Can you work these out from the model? Positions are in its coordinate system, mm. A direction names the side the tool comes from. Give positions to 0.01 mm unless a question says otherwise; leave off trailing zeros. Loops run counter-clockwise (first coordinate to the right, second up) from the corner with the lowest first, then second, coordinate; pieces in that order, holes last. Notation, with made-up numbers: (86, -14) - (129, -14) arc R13 cw to (129, 3) - close; hole circle Ø11 at (17.5, 57). An arc over 180 degrees is marked (long way). Answer as a JSON object with one key per item and string values.
```python
from build123d import *

# Parameters (mm, degrees)
IZIM1_W                     = 10
IZIM1_H                     = 20
Y_KSEKLIK_EKSTR_ZYON1_DEPTH = 150
BO_ALTMA1_T                 = -1
IZIM4_R                     = 2
KES_EKSTR_ZYON3_DEPTH       = 18


with BuildPart() as part:
    # Çizim1 → Yükseklik-Ekstrüzyon1 (new, symmetric)
    with BuildSketch(Plane.XY):
        Rectangle(IZIM1_W, IZIM1_H)
    extrude(amount=Y_KSEKLIK_EKSTR_ZYON1_DEPTH, both=True)

    # İç Boşaltma1
    bo_altma1_openings = [part.faces().sort_by_distance(p)[0] for p in [
        (0, 0, 150),
    ]]
    offset(amount=BO_ALTMA1_T, openings=bo_altma1_openings, kind=Kind.INTERSECTION)

    # Çizim4 → Kes-Ekstrüzyon3 (cut)
    with BuildSketch(Plane(origin=(5, 0, 0), x_dir=(0, 0, -1), z_dir=(1, 0, 0))):
        with Locations(Location((-99.95519869, 6.5, 0), (0, 0, 90))):
            Circle(IZIM4_R)
        with Locations(Location((-99.95519869, -6.5, 0), (0, 0, 90))):
            Circle(IZIM4_R)
    extrude(amount=-KES_EKSTR_ZYON3_DEPTH, mode=Mode.SUBTRACT)


solid = part.part
```
1) I'm going to push a flat-ended pin straight in: P1, Ø3.5, axis at y = 6.5, z = 99.96, coming from the +X side. Where does the tip first touch, or does it pass through?
Check sheet entries:
{"P1": "through"}
2) I need wall thicknesses on L1, parallel to Y at x = -0.25, z = -32.5; L2, parallel to X at y = -6.75, z = -80.5; L3, parallel to Z at x = 4.5, y = -6.5. Which ranges of each line are inside material? Lowest first, please.
Check sheet entries:
{"L1": "-10 to -9, 9 to 10", "L2": "-5 to -4, 4 to 5", "L3": "-150 to 97.96, 101.96 to 150"}
3) Imagine slicing it at A-A on x = -1.75. Write out the boundary of the cut face in (y, z), and give its area (3 significant figures).
Check sheet entries:
{"outline": "(-10, -150) - (10, -150) - (10, 150) - (9, 150) - (9, -149) - (-9, -149) - (-9, 150) - (-10, 150) - close", "area": "618 mm2"}
4) If we mould it in two halves opening along Y, with no side actions, what happens to faces 3 (the flat face through (0, 0, -150)), 4 (the flat face through (-4, 0, 3)), 5 (the flat face through (0, 9, 3)), 6 (the flat face through (0, 10, 2))? For each: released by +Y, released by -Y, zero draft, split by the parting line, or undercut.
Check sheet entries:
{"face 3": "zero draft", "face 4": "undercut", "face 5": "undercut", "face 6": "released by +Y"}
5) Imagine slicing it at B-B on z = 106.5. Write out the boundary of the cut face in (x, y), and give its area (3 significant figures).
Check sheet entries:
{"outline": "(-5, -10) - (5, -10) - (5, 10) - (-5, 10) - close; hole (-4, -9) - (4, -9) - (4, 9) - (-4, 9) - close", "area": "56.0 mm2"}
6) Which directions (+Z, -Z, +X, -X, +Y, -Y) give clear straight access to the entire face, cutting with the end or side of a thin tool? Please do faces 1 (the flat face through (0, -9, 3)), 2 (the flat face through (5, 0, 2)).
Check sheet entries:
{"face 1": "+Z", "face 2": "+Z, -Z, +X, +Y, -Y"}
